For this review, use the dimensioned drawing (mm, ordinates from the lowest corner) and the shaded views. A direction names the side the tool comes from. Round coordinates to 2 decimals unless told otherwise and drop trailing zeros. Loops run counter-clockwise (first coordinate to the right, second up) from the corner with the lowest first, then second, coordinate; pieces in that order, holes last. Notation, with made-up numbers: (83.25, -38) -> (135.25, -38) arc R19 ccw to (135.25, -13) -> close; hole circle Ø2 at (20.5, 36.25). An arc over 180 degrees is marked (long way). Write each question's results on one line, items separated by ' | '.
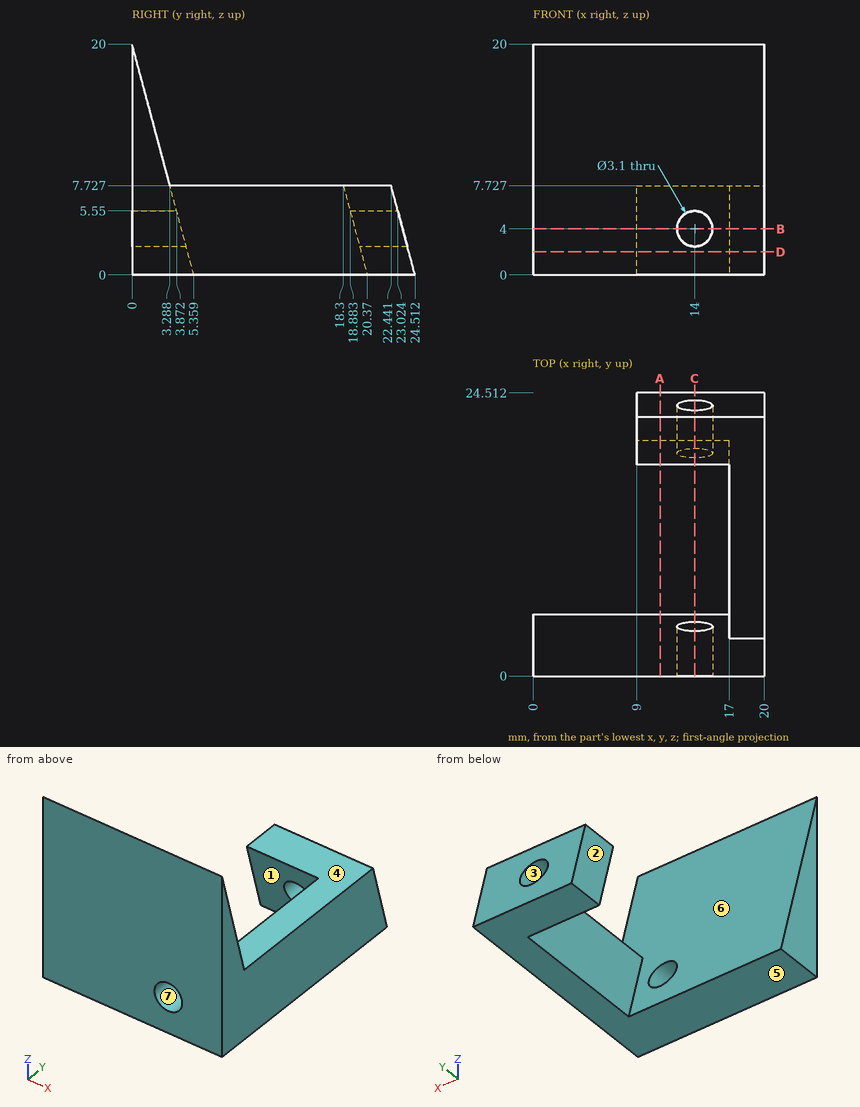
1. Consider section C-C (x = 14). Give the number of separate pieces and of enclosed holes in the cut face.
Values found:
separate pieces: 4 | enclosed holes: 0
2. Consider section D-D (z = 2). State the section outline as (x, y) points (1 decimal).
Values found:
outline: (0, 0) -> (20, 0) -> (20, 24) -> (9, 24) -> (9, 19.8) -> (17, 19.8) -> (17, 4.8) -> (0, 4.8) -> close
3. Draft analysis for pull direction Z (two halves, no side actions). For the marked faces 5, 6 and 7, state which applies: released by +Z, released by -Z, zero draft, split by the parting line, or undercut.
Values found:
face 5: released by -Z | face 6: released by +Z | face 7: undercut
4. Consider section B-B (z = 4). State the section outline as (x, y) points, plus the area to 3 significant figures.
Values found:
outline: (0, 0) -> (12.45, 0) -> (12.45, 4.29) -> (0, 4.29) -> close; (9, 19.3) -> (12.45, 19.3) -> (12.45, 23.44) -> (9, 23.44) -> close; (15.55, 0) -> (20, 0) -> (20, 23.44) -> (15.55, 23.44) -> (15.55, 19.3) -> (17, 19.3) -> (17, 4.29) -> (15.55, 4.29) -> close | area: 150 mm2
5. Tool access review of the marked faces 1, 2, 3 and 4: name each direction out of +Z, -Z, +X, -X, +Y, -Y from which nothing blocks a thin tool from reaching the whole face with its end or side.
Values found:
face 1: -Z, -X | face 2: +Z, -Z, -X, +Y | face 3: +Y, -Y | face 4: +Z, +X, -X, +Y
6. For pin 1 (3.5 mm diameter, centred on x = 14, z = 4, fed in from +Y); pin 2 (3 mm diameter, centred on x = 3, z = 10, fed in from +Y); pin 3 (2 mm diameter, centred on x = 4, z = 8.5, fed in from +Y), all flat-tipped, find the tip position at first contact; note any pin that passes through.
Values found:
pin 1: stops at y = 23.91 | pin 2: stops at y = 3.08 | pin 3: stops at y = 3.35
7. To check wall thickness, follow probe 1 along X at (y, z) = (1.5, 4); probe 2 along X at (y, z) = (20.55, 4); probe 3 along Z at (x, y) = (14, 22). State the ranges of each line that lie inside material, in increasing order.
Values found:
probe 1: x = 0 to 12.45, 15.55 to 20 | probe 2: x = 9 to 12.45, 15.55 to 20 | probe 3: z = 0 to 2.45, 5.55 to 7.73
8. Consider section A-A (x = 11). State the section outline as (y, z) points.
Values found:
outline: (0, 0) -> (5.36, 0) -> (0, 20) -> close; (18.3, 7.73) -> (20.37, 0) -> (24.51, 0) -> (22.44, 7.73) -> close
